For this review, take the finished solid that the model builds, in its own axes (mm). Coordinates: 2 decimals unless noted, no trailing zeros. Write each loop counter-clockwise with the first axis right and the second up, starting at its lowest first coordinate (ties: lowest second). Pieces come first, ordered by that corner, then holes.
Autodesk Inventor part; units mm, degrees
ref_plane "YZ Plane" through (0, 0, 0) normal (1, 0, 0) x (0, 1, 0)
ref_plane "XZ Plane" through (0, 0, 0) normal (0, 1, 0) x (-1, 0, 0)
ref_plane "XY Plane" through (0, 0, 0) normal (0, 0, 1) x (1, 0, 0)
sketch "Sketch1" plane through (0, 0, 0) normal (0, 1, 0) x (-1, 0, 0)
  line L0 (95.4024, 35.0012) -> (-95.4024, 35.0012)
  line L1 (-95.4024, 35.0012) -> (-95.4024, -35.0012)
  line L2 (-95.4024, -35.0012) -> (95.4024, -35.0012)
  line L3 (95.4024, -35.0012) -> (95.4024, 35.0012)
  line L4 (95.4024, 35.0012) -> (-95.4024, -35.0012) construction
  line L5 (-95.4024, 35.0012) -> (95.4024, -35.0012) construction
  circle A0 centre (82.7024, -22.3012) radius 3.302
  circle A1 centre (-82.7024, -22.3012) radius 3.302
  circle A2 centre (-82.7024, 22.3012) radius 3.302
  circle A3 centre (82.7024, 22.3012) radius 3.302
  line L6 (40.9111, -19.05) -> (-47.9889, -19.05) construction
  line L7 (40.9111, 19.05) -> (-47.9889, 19.05) construction
  circle A4 centre (23.8125, -19.05) radius 2.413
  circle A5 centre (-23.8125, -19.05) radius 2.413
  circle A6 centre (23.8125, 19.05) radius 2.413
  circle A7 centre (-23.8125, 19.05) radius 2.413
  point P0 (0, 0)
  dimension "d0" = 190.8048
  dimension "d1" = 70.0024
  dimension "d2" = 6.604
  dimension "d3" = 12.7
  dimension "d4" = 12.7
  dimension "d5" = 6.604
  dimension "d6" = 12.7
  dimension "d7" = 6.604
  dimension "d8" = 12.7
  dimension "d9" = 6.604
  dimension "d10" = 88.9
  dimension "d11" = 88.9
  dimension "d12" = 38.1
  dimension "d13" = 19.05
  dimension "d14" = 4.826
  dimension "d15" = 4.826
  dimension "d16" = 47.625
  dimension "d17" = 23.8125
  dimension "d18" = 4.826
  dimension "d19" = 4.826
extrude "Extrusion1" add sketch "Sketch1" along normal blind 6.35
properties part number "SequenceMachine_ManifoldPlate"
Q1. Add section A-A (x = 24.5). State the section outline as (y, z) points.
Ans:
outline: (0, -35) - (6.35, -35) - (6.35, -21.36) - (0, -21.36) - close; (0, -16.74) - (6.35, -16.74) - (6.35, 16.74) - (0, 16.74) - close; (0, 21.36) - (6.35, 21.36) - (6.35, 35) - (0, 35) - close
Q2. For probe 1 along X at (y, z) = (5.25, -22.5); probe 2 along X at (y, z) = (2, -21), list the stretches that pass through material, from the lowest coordinate up.
Ans:
probe 1: x = -95.4 to -86, -79.41 to 79.41, 86 to 95.4
probe 2: x = -95.4 to -85.74, -79.67 to -25.23, -22.39 to 22.39, 25.23 to 79.67, 85.74 to 95.4
Q3. Draft analysis for pull direction Z (two halves, no side actions). For faces 1 (the cylindrical face through (21.51, 3.13, -19.77)), 2 (the flat face through (1, 3, -35.001)), 3 (the flat face through (95.402, 3, 0)), state which applies: +Z half, -Z half, draft (parallel to the pull), parting line (faces both ways), or undercut.
Ans:
face 1: undercut
face 2: -Z half
face 3: draft
Q4. Add section B-B (y = 1.25). Give the number of separate pieces and of enclosed holes in the cut face, then the cut area to 3 significant figures.
Ans:
separate pieces: 1
enclosed holes: 8
area: 13,100 mm2
